Part model, mm, in its own coordinate system. A direction names the side the tool comes from. Round coordinates to 2 decimals unless told otherwise and drop trailing zeros. Loops run counter-clockwise (first coordinate to the right, second up) from the corner with the lowest first, then second, coordinate; pieces in that order, holes last. Notation, with made-up numbers: M 62.5,11 L 66.5,11 A13 cw 66.5,26 Z; hole C 41.25,83.25 d10. An arc over 180 degrees is marked long. Put each result on its own line as item: value. Start each with the question number.
1) Slice it at D-D on y = -34.5. Give the cut face in (x, z), then the cut area to 3 significant figures.
2) Slice it at A-A on x = 49. Give the cut face in (y, z).
3) Drop flat-ended pins along their axis: pin 1 Ø3.5 at (y, z) = (-29.5, -13) entering from -X; pin 2 Ø0.5 at (x, z) = (60.5, -26) entering from +Y; pin 3 Ø1.1 at (x, z) = (60.5, -3) entering from +Y; pin 4 Ø1.5 at (x, y) = (43, -15.5) entering from -Z. Give the stop position or say it passes through.
4) Which spindle directions (+Z, -Z, +X, -X, +Y, -Y) get a long thin tool onto all of the face, cutting with end or side? Do faces 5 (the flat face through (27.4, -25, -14.8)), 6 (the flat face through (34, -18, -15)), 7 (the flat face through (49, -24, 10)). Say none if no direction does.
5) Pull direction Z, two halves, no side cores. Call faces 1 (the cylindrical face through (54.08, -12.13, -17.32)), 2 (the flat face through (27.93, -36.99, -36.01)), 3 (the flat face through (27.594, -30.67, -1.066)), 4 (the flat face through (54, 0, -15)): +Z half, -Z half, draft (parallel to the pull), parting line (faces both ways), or undercut.
6) Probe line 1 along Y through (x, z) = (56, -15); line 2 along Z through (x, y) = (54, -10); line 3 along X through (y, z) = (-6.5, -7.5). List the from-to ranges inside material, lowest first.
7) Slice it at B-B on z = -15. Give the cut face in (x, y), then the cut area to 3 significant figures.
8) Slice it at C-C on y = -8.5. Give the cut face in (x, z).
```python
from build123d import *

# Parameters (mm, degrees)
SKETCH047_R     = 2
PAD012_DEPTH    = 25
SKETCH048_R     = 3.15
POCKET030_DEPTH = 40.001
SKETCH049_W     = 28
SKETCH049_H     = 50
POCKET031_DEPTH = 18
PAD013_DEPTH    = 12.5
SKETCH051_W     = 20
SKETCH051_H     = 8
PAD014_DEPTH    = 1
CHAMFER009_SIZE = 0.99
CHAMFER010_SIZE = 1
CHAMFER011_SIZE = 5


with BuildPart() as part:
    # Sketch047 → Pad012 (new body)
    with BuildSketch(Plane.XZ):
        Polygon((0, 0), (-30, 0), (-40, 15), (-40, 35), (-30, 50), (0, 50), align=None)
        with Locations((-35, 25)):
            Circle(SKETCH047_R, mode=Mode.SUBTRACT)
    extrude(amount=-PAD012_DEPTH)

    # Sketch048 (on Face6 of Pad012) → Pocket030 (cut, through all)
    with BuildSketch(Plane(origin=(0, 0, 0), x_dir=(0, 0, 1), z_dir=(1, 0, 0))):
        with Locations((25, -15)):
            Circle(SKETCH048_R)
    extrude(amount=-POCKET030_DEPTH, mode=Mode.SUBTRACT)

    # Sketch049 (on Face5 of Pocket030) → Pocket031 (cut)
    with BuildSketch(Plane(origin=(0, 25, 0), x_dir=(1, 0, 0), z_dir=(0, 1, 0))):
        with Locations((-26, -25)):
            Rectangle(SKETCH049_W, SKETCH049_H)
    extrude(amount=-POCKET031_DEPTH, mode=Mode.SUBTRACT)

    # Sketch050 (on Face2 of Pocket031) → Pad013 (join)
    with BuildSketch(Plane.XZ):
        Polygon((-34.891667, 42.6625), (-29.85, 35.1), (-29.85, 14.9), (-34.891667, 7.3375), (-30, 0), (0, 0), (0, 50), (-30, 50), align=None)
    extrude(amount=PAD013_DEPTH)

    # Sketch051 (on Face14 of Pad013) → Pad014 (join)
    with BuildSketch(Plane(origin=(0, 0, 0), x_dir=(0, 0, 1), z_dir=(1, 0, 0))):
        with Locations((10, -15)):
            Rectangle(SKETCH051_W, SKETCH051_H)
        with Locations((40, -15)):
            Rectangle(SKETCH051_W, SKETCH051_H)
    extrude(amount=PAD014_DEPTH)

    # Chamfer009
    chamfer009_edges = [part.edges().sort_by_distance(p)[0] for p in [
        (1, 11, 40),
        (1, 11, 10),
    ]]
    chamfer(chamfer009_edges, length=CHAMFER009_SIZE)

    # Chamfer010
    chamfer010_edges = [part.edges().sort_by_distance(p)[0] for p in [
        (-32.370833, -12.5, 38.88125),
        (-29.85, -12.5, 25),
        (-32.370833, -12.5, 11.11875),
        (-32.445833, -12.5, 3.66875),
        (-15, -12.5, 0),
        (0, -12.5, 25),
        (-15, -12.5, 50),
        (-32.445833, -12.5, 46.33125),
    ]]
    chamfer(chamfer010_edges, length=CHAMFER010_SIZE)

    # Chamfer011
    chamfer011_edges = [part.edges().sort_by_distance(p)[0] for p in [
        (-6, 25, 50),
        (-6, 25, 0),
    ]]
    chamfer(chamfer011_edges, length=CHAMFER011_SIZE)


with BuildPart() as part_1:
    # Body004 placement: moved
    add(part.part.moved(Location((60, -25, -40))))


solid = part_1.part
```
Recorded:
1. outline: M 25.11,-32.66 L 30,-40 L 60,-40 L 60,10 L 30,10 L 25.11,2.66 L 30.15,-4.9 L 30.15,-25.1 Z
1. area: 1,570 mm2
2. outline: M -37.5,-39 L -36.5,-40 L -5,-40 L 0,-35 L 0,5 L -5,10 L -36.5,10 L -37.5,9 Z; hole C -10,-15 d6.3
3. pin 1: stops at x = 30.15
3. pin 2: stops at y = -6
3. pin 3: stops at y = 0
3. pin 4: passes through
4. face 5: -X, -Y
4. face 6: +Z, -Z, -X, +Y
4. face 7: +Z, +X, -X, +Y, -Y
5. face 1: undercut
5. face 2: -Z half
5. face 3: undercut
5. face 4: draft
6. line 1: y = -37.5 to -13.15, -6.85 to 0
6. line 2: z = -40 to -18.15, -11.85 to 10
6. line 3: x = 48 to 61
7. outline: M 20,-25 L 23,-25 L 23,-18 L 20,-18 Z; M 27,-25 L 30.15,-25 L 30.15,-36.5 L 31.15,-37.5 L 59,-37.5 L 60,-36.5 L 60,-13.15 L 48,-13.15 L 48,-18 L 27,-18 Z; M 48,-6.85 L 60,-6.85 L 60,0 L 48,0 Z
7. area: 765 mm2
8. outline: M 48,-40 L 61,-40 L 61,-20 L 60,-20 L 60,-17.77 L 48,-17.77 Z; M 48,-12.23 L 60,-12.23 L 60,-10 L 61,-10 L 61,10 L 48,10 Z
